Autodesk Inventor part; units mm, degrees
ref_plane "YZ Plane" through (0, 0, 0) normal (1, 0, 0) x (0, 1, 0)
ref_plane "XZ Plane" through (0, 0, 0) normal (0, 1, 0) x (-1, 0, 0)
ref_plane "XY Plane" through (0, 0, 0) normal (0, 0, 1) x (1, 0, 0)
sketch "Sketch1" plane through (0, 0, 0) normal (0, 0, 1) x (1, 0, 0)
  line L0 (-6.0944, 0.2158) -> (-25.1502, 0.2158)
  line L1 (-25.1502, 0.2158) -> (-25.1502, -4.7842)
  line L2 (-25.1502, -4.7842) -> (-5.1501, -4.7842)
  line L3 (-5.1501, -4.7842) -> (-5.0826, -24.7842)
  line L4 (-5.0826, -24.7842) -> (-0.0826, -24.7842)
  line L5 (-0.0826, -24.7842) -> (-0.1467, -5.8041)
  line L6 (-6.0944, 0.2158) -> (16.1426, 22.6034)
  line L7 (22.0903, 16.5836) -> (-0.1467, -5.8041)
  circle A0 centre (21.0114, 21.4658) radius 1.85
  arc A1 (22.0903, 16.5836) -> (16.1426, 22.6034) centre (21.0114, 21.4658) ccw
  dimension "d0" = 20
  dimension "d1" = 20
  dimension "d2" = 5
  dimension "d3" = 5
  dimension "d7" = 26.25
  dimension "d8" = 26.25
  dimension "d9" = 3.7
  dimension "d18" = 5
  dimension "d19" = 135
extrude "Extrusion1" add sketch "Sketch1" along normal blind 30
ref_plane "Work Plane1" through (0, 0, 24) normal (0, 0, 1) x (1, 0, 0)
sketch "Sketch3" plane through (0, 0, 24) normal (0, 0, 1) x (1, 0, 0)
  circle A0 centre (21.0114, 21.4658) radius 1.85
  circle A1 centre (21.0114, 21.4658) radius 12.5
  point P0 (0, 0)
  dimension "d13" = 25
extrude "Extrusion3" cut sketch "Sketch3" against normal blind 18
sketch "Sketch5" plane through (0, 0, 0) normal (0, 0, -1) x (-1, 0, 0)
  circle A0 centre (-21.0114, 21.4658) radius 1.85
  line L0 (25.1502, -4.7842) -> (25.1502, 0.2158)
  line L1 (25.1502, 0.2158) -> (6.0944, 0.2158)
  line L2 (6.0944, 0.2158) -> (-16.1426, 22.6034)
  arc A1 (-16.1426, 22.6034) -> (-22.0903, 16.5836) centre (-21.0114, 21.4658) ccw
  line L3 (-22.0903, 16.5836) -> (0.1467, -5.8041)
  line L4 (0.1467, -5.8041) -> (0.0826, -24.7842)
  line L5 (0.0826, -24.7842) -> (5.0826, -24.7842)
  line L6 (5.0826, -24.7842) -> (5.1501, -4.7842)
  line L7 (5.1501, -4.7842) -> (25.1502, -4.7842)
  line L8 (0.1467, -5.8041) -> (6.0944, 0.2158)
  point P0 (0, 0)
extrude "Extrusion5" add sketch "Sketch5" along normal blind 25 contours L7 L6 L5 L4 L8 L1 L0
sketch "Sketch8" plane through (-5.0826, -24.7842, -25) normal (-1, -0.0034, 0) x (0, 0, 1)
  circle A0 centre (10, 10) radius 2.25
  line L0 (55, 0) -> (0, 0)
  line L1 (0, 0) -> (0, 20.0001)
  circle A1 centre (25, 10) radius 2.25
  point P0 (25, 24.7669)
  dimension "d40" = 4.5
  dimension "d41" = 10
  dimension "d42" = 10
  dimension "d43" = 4.5
  dimension "d44" = 10
  dimension "d45" = 15
sketch "Sketch9" plane through (-25.1502, 0.2158, 30) normal (0, 1, 0) x (1, 0, 0)
  circle A0 centre (10, 45) radius 2.25
  circle A1 centre (10, 30) radius 2.25
  line L0 (0, 55) -> (19.0558, 55)
  line L1 (0, 0) -> (0, 55)
  point P0 (25.1502, 30)
  dimension "d46" = 10
  dimension "d47" = 10
  dimension "d48" = 10
  dimension "d49" = 15
  dimension "d50" = 4.5
  dimension "d51" = 4.5
extrude "Extrusion8" cut sketch "Sketch9" against normal mid plane 20
extrude "Extrusion9" cut sketch "Sketch8" against normal blind 20
sketch "Sketch10" plane through (0, 0, 30) normal (0, 0, 1) x (1, 0, 0)
  line L0 (-3.9108, 3.9108) -> (4.5333, -4.5333)
  line L1 (4.5333, -4.5333) -> (4.5333, -31.01)
  line L2 (4.5333, -31.01) -> (-28.169, -31.01)
  line L3 (-28.169, -31.01) -> (-28.169, 3.9108)
  line L4 (-28.169, 3.9108) -> (-3.9108, 3.9108)
  point P0 (0, 0)
  dimension "d56" = 135
  dimension "d57" = 0
extrude "Extrusion10" cut sketch "Sketch10" against normal blind 15
equation "\"d43\" = d40"
equation "\"d44\" = d41"
equation "\"RodDiameter\" = 8"
equation "\"VerticalBearingOD\" = 16"
equation "\"PrintingClearance\" = 0.2"
equation "\"TubeID\" = 18"
properties part number "PulleyHolderXY"
Design review of the part built by this model. Coordinates are the model's own, in mm. A direction names the side the tool comes from. Give positions to 0.01 mm unless a question says otherwise; leave off trailing zeros. Loops run counter-clockwise (first coordinate to the right, second up) from the corner with the lowest first, then second, coordinate; pieces in that order, holes last. Notation, with made-up numbers: (43, 11.5) - (98, 11.5) arc R20 cw to (98, 27.5) - close; hole circle Ø2 at (70, 40.5). An arc over 180 degrees is marked (long way). Use CSV: the item, a comma, the result in double quotes. Start each with the question number.
1. Add section A-A (z = 9.5). State the section outline as (x, y) points, plus the area to 3 significant figures.
2. Add section D-D (x = 13.5). State the section outline as (y, z) points, plus the area to 3 significant figures.
3. Machinability: for faces 1 (the flat face through (-15, -4.784, -5)), 2 (the flat face through (-8.1, -4.5, 15)), 3 (the flat face through (18, 18, 24)), 4 (the flat face through (-16, 0.216, -5)), 5 (the cylindrical face through (-15.638, -2.249, -12.804)), which of the approach directions +Z, -Z, +X, -X, +Y, -Y give a long, thin tool a straight path to every point of the face, cutting with its end or side? Answer none if there is none.
4. Add section C-C (z = -15). State the section outline as (x, y) points, plus the area to 3 significant figures.
5. Add section B-B (y = 17.5). State the section outline as (x, z) points, plus the area to 3 significant figures.
6. Draft analysis for pull direction Z (two halves, no side actions). For faces 6 (the flat face through (-3, -24.784, -5)), 7 (the cylindrical face through (12.1, 12.7, 15.1)), 8 (the flat face through (-4, -8, -25)), state which applies: released by +Z, released by -Z, zero draft, split by the parting line, or undercut.
7. Insertion check: P1, Ø8.5, axis at x = -11.5, y = -14, coming from the +Z side; P2, Ø1, axis at x = -11.5, z = 6, coming from the +Y side; P3, Ø22, axis at x = -14.5, z = -6, coming from the -Y side; P4, Ø18, axis at x = 15, y = 18, coming from the -Z side. Each pin has a flat end and moves straight along its axis. Give the tip position at first contact, or say it passes through.
8. Wall thickness on L1, parallel to Y at x = -14.5, z = 7; L2, parallel to Z at x = 19, y = 24.5; L3, parallel to X at y = -1, z = -15: over which ranges is each line inside the solid? List them lowest first.
Results found:
1,outline,"(-25.15, -4.78) - (-5.15, -4.78) - (-5.08, -24.78) - (-0.08, -24.78) - (-0.15, -5.8) - (15.7, 10.15) arc R12.5 cw to (9.71, 16.13) - (-6.09, 0.22) - (-25.15, 0.22) - close"
1,area,"393 mm²"
2,outline,"(7.94, 0) - (19.94, 0) - (19.94, 6) - (11.47, 6) - (11.47, 24) - (19.94, 24) - (19.94, 30) - (7.94, 30) - close"
2,area,"208 mm²"
3,face 1,"+Z, -Z, -X, -Y"
3,face 2,"+Z, -X, -Y"
3,face 3,"+X, +Y"
3,face 4,"+Z, -Z, -X, +Y"
3,face 5,"+Y, -Y"
4,outline,"(-25.15, -4.78) - (-17.4, -4.78) - (-17.4, 0.22) - (-25.15, 0.22) - close; (-12.9, -4.78) - (-5.15, -4.78) - (-5.12, -12.53) - (-0.12, -12.52) - (-0.15, -5.8) - (-6.09, 0.22) - (-12.9, 0.22) - close; (-5.11, -17.03) - (-5.08, -24.78) - (-0.08, -24.78) - (-0.11, -17.02) - close"
4,area,"162 mm²"
5,outline,"(11.07, 0) - (24.06, 0) - (24.06, 6) - (11.07, 6) - close; (11.07, 24) - (24.06, 24) - (24.06, 30) - (11.07, 30) - close"
5,area,"156 mm²"
6,face 6,"zero draft"
6,face 7,"undercut"
6,face 8,"released by -Z"
7,P1,"passes through"
7,P2,"stops at y = 0.22"
7,P3,"stops at y = -24.78"
7,P4,"stops at z = 0"
8,L1,"y = -4.78 to 0.22"
8,L2,"z = 0 to 6, 24 to 30"
8,L3,"x = -25.15 to -17.4, -12.9 to -4.89"
